The figure shows three views and two pictorial views of one solid part (mm, origin at its lowest corner). Answer the questions. Coordinates: 2 decimals unless noted, no trailing zeros. Loops run counter-clockwise (first coordinate to the right, second up) from the corner with the lowest first, then second, coordinate; pieces in that order, holes last. Notation, with made-up numbers: M -14.75,-28 L 16.25,-28 A15 cw 16.25,-15 Z; hole C 25,1.5 d10. An arc over 180 degrees is marked long. Return JSON: item names as keys, results as strings. Group by question number.
1. Section B-B (z = 0.8) is taken. Write down the section's boundary in (x, y).
2. Section D-D (x = 21) is taken. Write down the section's boundary in (y, z) (3 decimals), then the cut area to 3 significant figures.
3. Straight lines are drawn through the part: L1, parallel to Y at x = 37.5, z = 1.25; L2, parallel to Y at x = 66, z = 1; L3, parallel to X at y = 55, z = 3.3. For each, find the intervals that lie inside material, in ascending order. Write a range as from..to.
4. Section C-C (y = 53.75) is taken. Write down the section's boundary in (x, z).
5. Given P1, Ø2, axis at x = 37.5, y = 70, coming from the -Z side; P2, Ø5.5, axis at x = 65.65, y = 53.75, coming from the +Z side, each flat-ended and moving along its own axis, determine where each tip first touches the part or whether it passes through.
6. Section A-A (y = 70) is taken. Write down the section's boundary in (x, z).
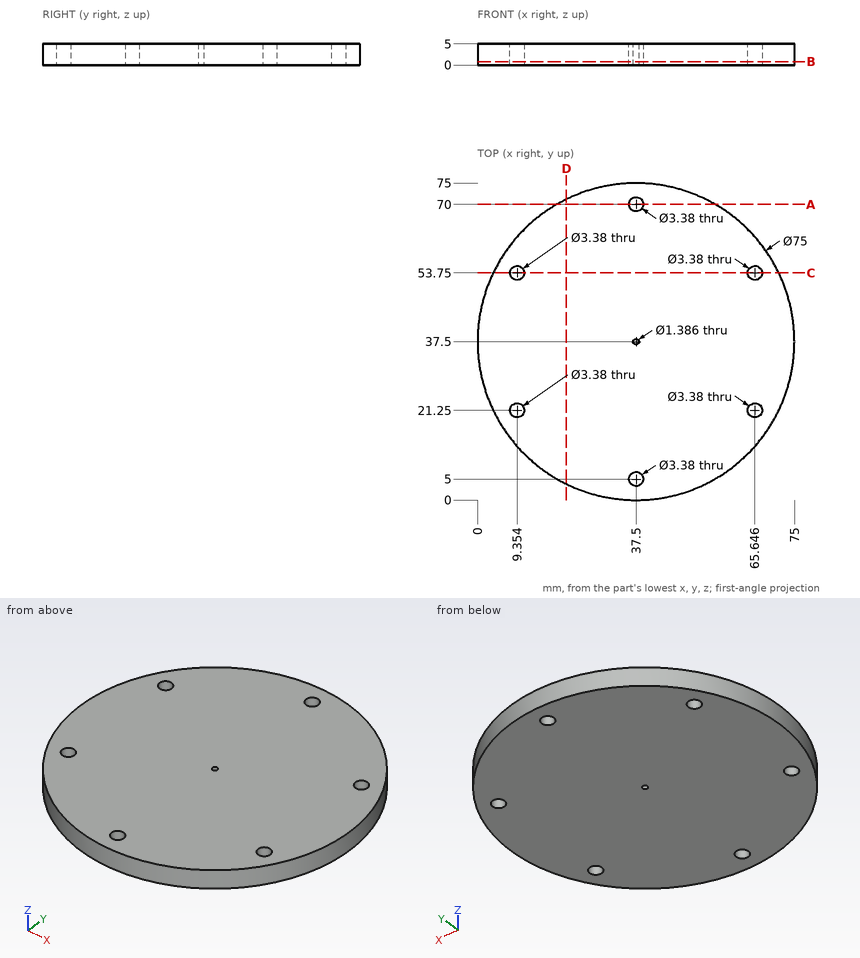
Worked out:
{
 "1": {"outline": "C 37.5,37.5 d75; hole C 9.35,21.25 d3.38; hole C 9.35,53.75 d3.38; hole C 37.5,5 d3.38; hole C 37.5,70 d3.38; hole C 37.5,37.5 d1.39; hole C 65.65,21.25 d3.38; hole C 65.65,53.75 d3.38"},
 "2": {"outline": "M 3.825,0 L 71.175,0 L 71.175,5 L 3.825,5 Z", "area": "337 mm^2"},
 "3": {"L1": "0..3.31, 6.69..36.81, 38.19..68.31, 71.69..75", "L2": "13.13..19.6, 22.9..52.1, 55.4..61.87", "L3": "4.33..8.22, 10.49..64.51, 66.78..70.67"},
 "4": {"outline": "M 3.7,0 L 7.66,0 L 7.66,5 L 3.7,5 Z; M 11.04,0 L 63.96,0 L 63.96,5 L 11.04,5 Z; M 67.34,0 L 71.3,0 L 71.3,5 L 67.34,5 Z"},
 "5": {"P1": "through", "P2": "z = 5"},
 "6": {"outline": "M 18.79,0 L 35.81,0 L 35.81,5 L 18.79,5 Z; M 39.19,0 L 56.21,0 L 56.21,5 L 39.19,5 Z"}
}
